Design review of the part built by this model. Coordinates are the model's own, in mm. A direction names the side the tool comes from. Coordinates: 2 decimals unless noted, no trailing zeros. Write each loop counter-clockwise with the first axis right and the second up, starting at its lowest first coordinate (ties: lowest second). Pieces come first, ordered by that corner, then holes. Notation, with made-up numbers: (-33, 51.25) -> (-28, 51.25) arc R20 ccw to (-28, 66.25) -> close; hole circle Ø2 at (-1, 37). An arc over 180 degrees is marked (long way). Return JSON: item names as keys, results as strings. Group by question number.
from build123d import *

# Parameters (mm, degrees)
F0_W     = 7.2136
F0_H     = 10.287
F0_H_2   = 17.2237775958
F2_R     = 1.5875
F3_R     = 0.79375
F4_SIZE2 = 6.35
F4_SIZE  = 1.5748


with BuildPart() as f1:
    # F0 (on Right) → F1 (revolve)
    with BuildSketch(Plane.YZ):
        with Locations((3.6068, 30.5435)):
            Rectangle(F0_W, F0_H)
        with Locations((3.6068, 16.7881112021)):
            Rectangle(F0_W, F0_H_2)
        Polygon((7.2136, 8.1762224042), (0, 8.1762224042), (0, 7.9375), (29.4386, 7.9375), (29.4386, 25.4), (7.2136, 25.4), align=None)
    revolve(axis=Axis((0, 15.9048408099, 0), (0, 1, 0)))

    # F2
    f2_edges = [f1.edges().sort_by_distance(p)[0] for p in [
        (0, 7.2136, -25.4),
    ]]
    fillet(f2_edges, radius=F2_R)

    # F3
    f3_edges = [f1.edges().sort_by_distance(p)[0] for p in [
        (0, 29.4386, -25.4),
    ]]
    fillet(f3_edges, radius=F3_R)

    # F4
    f4_edges = [f1.edges().sort_by_distance(p)[0] for p in [
        (0, 0, -35.687),
        (0, 7.2136, -35.687),
    ]]
    f4_side = f1.faces().sort_by_distance((0, 3.6068, -35.687))[0]
    chamfer(f4_edges, length=F4_SIZE, length2=F4_SIZE2, reference=f4_side)


solid = f1.part
Q1. We need section C-C on y = 3.75. Write out the cut boundary in (x, z) (1 decimal).
Q2. Wall thickness on L1, parallel to X at y = 15, z = 0; L2, parallel to Z at x = -7, y = 8.25; L3, parallel to X at y = 13.5, z = -6: over which ranges is each line inside the solid? List them lowest first.
Q3. For faces 1 (the cylindrical face through (-24.796, 18.584, -5.506)), 2 (the flat face through (-6, 0, 6)), list the 3-axis set-ups (+Z, -Z, +X, -X, +Y, -Y) from which the entire face can be reached by the end or side of a thin tool; tool diameter is ignored.
Q4. We need section B-B on x = 0. Write out the cut boundary in (y, z) (1 decimal).
Q5. For P1, Ø10, axis at x = -3.5, y = 23, coming from the +Z side; P2, Ø2, axis at y = 25, z = 4, coming from the +X side; P3, Ø1.5, axis at x = -18, z = -21.5, coming from the +Y side, all flat-tipped, find the tip position at first contact; note any pin that passes through.
Q6. The part is to be moulded in two halves that separate along X. For faces 3 (the flat face through (-24, 7.214, -13)), 4 (the cylindrical face through (-7.75, 14.93, -1.72)), 5 (the conical face through (-28.94, 7.137, -6.427)), say which applies: +X half, -X half, draft (parallel to the pull), parting line (faces both ways), or undercut.
Q7. We need section A-A on z = 0. Write out the cut boundary in (x, y) (1 decimal).
Findings below:
{
 "1": {"outline": "circle Ø71.4 at (0, 0); hole circle Ø15.9 at (0, 0)"},
 "2": {"L1": "x = -25.4 to -7.94, 7.94 to 25.4", "L2": "z = -24.52 to -3.74, 3.74 to 24.52", "L3": "x = -24.68 to -5.2, 5.2 to 24.68"},
 "3": {"face 1": "+Y", "face 2": "+Z, -Z, +X, -X, -Y"},
 "4": {"outline": "(0, -29.3) -> (1.6, -35.7) -> (5.6, -35.7) -> (7.2, -29.3) -> (7.2, -27) arc R1.6 cw to (8.8, -25.4) -> (28.6, -25.4) arc R0.8 ccw to (29.4, -24.6) -> (29.4, -7.9) -> (0, -7.9) -> close; (0, 7.9) -> (29.4, 7.9) -> (29.4, 24.6) arc R0.8 ccw to (28.6, 25.4) -> (8.8, 25.4) arc R1.6 cw to (7.2, 27) -> (7.2, 29.3) -> (5.6, 35.7) -> (1.6, 35.7) -> (0, 29.3) -> close"},
 "5": {"P1": "stops at z = 25.4", "P2": "stops at x = 25.22", "P3": "stops at y = 7.21"},
 "6": {"face 3": "draft", "face 4": "undercut", "face 5": "parting line"},
 "7": {"outline": "(-35.7, 1.6) -> (-29.3, 0) -> (-7.9, 0) -> (-7.9, 29.4) -> (-24.6, 29.4) arc R0.8 ccw to (-25.4, 28.6) -> (-25.4, 8.8) arc R1.6 cw to (-27, 7.2) -> (-29.3, 7.2) -> (-35.7, 5.6) -> close; (7.9, 0) -> (29.3, 0) -> (35.7, 1.6) -> (35.7, 5.6) -> (29.3, 7.2) -> (27, 7.2) arc R1.6 cw to (25.4, 8.8) -> (25.4, 28.6) arc R0.8 ccw to (24.6, 29.4) -> (7.9, 29.4) -> close"}
}
